```python
from build123d import *

# Parameters (mm, degrees)
SKETCH1_W             = 130
SKETCH1_H             = 93
BOSS_EXTRUDE1_DEPTH   = 5
SKETCH2_R             = 5.75
BOSS_EXTRUDE2_DEPTH   = 21.5
BOSS_EXTRUDE2_2_DEPTH = 21.5
SKETCH2_W             = 11.5
SKETCH2_H             = 11.5
BOSS_EXTRUDE2_3_DEPTH = 21.5
BOSS_EXTRUDE2_4_DEPTH = 21.5
SKETCH3_W             = 11.5
SKETCH3_H             = 19.25
SKETCH3_W_2           = 15.75
SKETCH3_H_2           = 11.5
BOSS_EXTRUDE3_DEPTH   = 5


with BuildPart() as part:
    # Sketch1 → Boss-Extrude1 (new body)
    with BuildSketch(Plane.XY):
        Rectangle(SKETCH1_W, SKETCH1_H)
    extrude(amount=BOSS_EXTRUDE1_DEPTH)



with BuildPart() as body_2:
    # Sketch2 → Boss-Extrude2 (new body)
    with BuildSketch(Plane.XY.offset(5)):
        with Locations((0, 60)):
            Circle(SKETCH2_R)
    extrude(amount=BOSS_EXTRUDE2_DEPTH)


with BuildPart() as body_3:
    # Sketch2 → Boss-Extrude2 2 (new body)
    with BuildSketch(Plane.XY.offset(5)):
        with Locations((75, 0)):
            Circle(SKETCH2_R)
    extrude(amount=BOSS_EXTRUDE2_2_DEPTH)


with BuildPart() as body_4:
    # Sketch2 → Boss-Extrude2 3 (new body)
    with BuildSketch(Plane.XY.offset(5)):
        with Locations((-75, 0)):
            Rectangle(SKETCH2_W, SKETCH2_H)
    extrude(amount=BOSS_EXTRUDE2_3_DEPTH)


with BuildPart() as body_5:
    # Sketch2 → Boss-Extrude2 4 (new body)
    with BuildSketch(Plane.XY.offset(5)):
        with Locations((0, -60)):
            Rectangle(SKETCH2_W, SKETCH2_H)
    extrude(amount=BOSS_EXTRUDE2_4_DEPTH)


with BuildPart() as part_1:
    add(part.part)

    add(body_2.part)  # Boss-Extrude3 merges body 2

    add(body_3.part)  # Boss-Extrude3 merges body 3

    add(body_4.part)  # Boss-Extrude3 merges body 4

    add(body_5.part)  # Boss-Extrude3 merges body 5
    # Sketch3 → Boss-Extrude3 (add)
    with BuildSketch(Plane(origin=(0, 0, 0), x_dir=(-1, 0, 0), z_dir=(0, 0, -1))):
        with Locations((0, 56.125)):
            Rectangle(SKETCH3_W, SKETCH3_H)
        with Locations((-72.875, 0)):
            Rectangle(SKETCH3_W_2, SKETCH3_H_2)
        with Locations((0, -56.125)):
            Rectangle(SKETCH3_W, SKETCH3_H)
        with Locations((72.875, 0)):
            Rectangle(SKETCH3_W_2, SKETCH3_H_2)
    extrude(amount=-BOSS_EXTRUDE3_DEPTH)


solid = part_1.part
```
Build history of the part. All positions in model axes, mm. A direction names the side the tool comes from. Give positions to 0.01 mm unless a question says otherwise; leave off trailing zeros. Loops run counter-clockwise (first coordinate to the right, second up) from the corner with the lowest first, then second, coordinate; pieces in that order, holes last.
Item 1: Pull direction Y, two halves, no side cores. Call faces 1 (the face through (0, -54.25, 16)), 2 (the face through (69.256, 0.253, 15.599)), 3 (the face through (3.09, 64.85, 15.6)), 4 (the face through (-80.75, 0, 13)): released by +Y, released by -Y, zero draft, split by the parting line, or undercut.
Answers follow:
face 1: undercut
face 2: split by the parting line
face 3: undercut
face 4: zero draft
Item 2: Slice it at C-C, the plane x = -3.5. List the corners of the cut face in (y, z).
Answers follow:
outline: (-65.75, 0) - (65.75, 0) - (65.75, 5) - (64.56, 5) - (64.56, 26.5) - (55.44, 26.5) - (55.44, 5) - (-54.25, 5) - (-54.25, 26.5) - (-65.75, 26.5) - close
Item 3: Slice it at D-D, the plane x = 29. List the corners of the cut face in (y, z).
Answers follow:
outline: (-46.5, 0) - (46.5, 0) - (46.5, 5) - (-46.5, 5) - close
Item 4: Drill centre lines: line 1 (Z direction, x = 22, y = 31); line 2 (Y direction, x = -55, z = 4.5); line 3 (X direction, y = 2, z = 11). Where is each one in solid material? Low to high.
Answers follow:
line 1: z = 0 to 5
line 2: y = -46.5 to 46.5
line 3: x = -80.75 to -69.25, 69.61 to 80.39
Item 5: Slice it at A-A, the plane z = 6.75. List the corners of the cut face in (x, y), and give its area (3 significant figures).
Answers follow:
outline: (-80.75, -5.75) - (-69.25, -5.75) - (-69.25, 5.75) - (-80.75, 5.75) - close; (-5.75, -65.75) - (5.75, -65.75) - (5.75, -54.25) - (-5.75, -54.25) - close; circle Ø11.5 at (0, 60); circle Ø11.5 at (75, 0)
area: 472 mm2
Item 6: Slice it at B-B, the plane y = -15. List the corners of the cut face in (x, z).
Answers follow:
outline: (-65, 0) - (65, 0) - (65, 5) - (-65, 5) - close
Item 7: Which spindle directions (+Z, -Z, +X, -X, +Y, -Y) get a long thin tool onto all of the face, cutting with end or side? Do faces 5 (the face through (35, 46.5, 2)), 6 (the face through (5.75, -58, 10)), 7 (the face through (-65, 26, 2)), 8 (the face through (-36, -46.5, 2)), 9 (the face through (80, -4, 5)). Say none if no direction does.
Answers follow:
face 5: +Z, -Z, +X, +Y
face 6: +Z, -Z, +X, -Y
face 7: +Z, -Z, -X, +Y
face 8: +Z, -Z, -X, -Y
face 9: +Z, +X, -Y
Item 8: Flat gauge pins, fed straight in: pin 1 (2.5 mm diameter, centred on y = 56, z = 1.5, fed in from +X); pin 2 (2.5 mm diameter, centred on x = -39, z = 3.5, fed in from +Y); pin 3 (10 mm diameter, centred on y = 6.5, z = 20, fed in from +X). Where does each tip first touch, or does it go through?
Answers follow:
pin 1: stops at x = 5.75
pin 2: stops at y = 46.5
pin 3: stops at x = 80.55
